```python
from build123d import *

# Parameters (mm, degrees)
SKETCH_1_W          = 95.5
SKETCH_1_H          = 95.5
EXTRUDE_1_DEPTH     = 7
CUT_EXTRUDE_1_DEPTH = 68.890536896
FILLET_2_R          = 15
SKETCH_3_R          = 75
EXTRUDE_2_DEPTH     = 2
CHAMFER_1_SIZE      = 7
FILLET_1_R          = 1
SKETCH_5_R          = 1.6
CUT_EXTRUDE_2_DEPTH = 107.296754489
SKETCH_6_W          = 42
SKETCH_6_H          = 42
CUT_EXTRUDE_3_DEPTH = 107.447170066
SKETCH_7_R          = 1.6
CUT_EXTRUDE_4_DEPTH = 107.447170066
CUT_EXTRUDE_5_DEPTH = 107.447170066
CUT_EXTRUDE_6_DEPTH = 0.5
SKETCH_10_W         = 12
SKETCH_10_H         = 12
CUT_EXTRUDE_7_DEPTH = 107.447170066
SKETCH_11_W         = 42
SKETCH_11_H         = 42
EXTRUDE_4_DEPTH     = 9
FILLET_3_R          = 2
SKETCH_12_W         = 41.3
SKETCH_12_H         = 41.3
CUT_EXTRUDE_8_DEPTH = 107.447170066
FILLET_4_R          = 5
SKETCH_13_R         = 3.25
CUT_EXTRUDE_9_DEPTH = 2


with BuildPart() as part:
    # ｽｹｯﾁ1 → ﾎﾞｽ - 押し出し1 (new body)
    with BuildSketch(Plane.XY):
        Rectangle(SKETCH_1_W, SKETCH_1_H)
    extrude(amount=EXTRUDE_1_DEPTH)

    # ｽｹｯﾁ2 → ｶｯﾄ - 押し出し1 (cut, through all)
    with BuildSketch(Plane.XY.offset(7)):
        Polygon((-16, 47.75), (-20, 20), (-47.75, 16), (-47.75, 47.75), align=None)
        Polygon((-16, -47.75), (-20, -20), (-47.75, -16), (-47.75, -47.75), align=None)
    cut_extrude_1 = extrude(amount=-CUT_EXTRUDE_1_DEPTH, mode=Mode.SUBTRACT)

    # ﾐﾗｰ1: ｶｯﾄ - 押し出し1 across plane
    add(cut_extrude_1.mirror(Plane(origin=(0, 0, 0), x_dir=(0, 0, 1), z_dir=(1, 0, 0))), mode=Mode.SUBTRACT)

    # ﾌｨﾚｯﾄ2
    fillet_2_edges = [part.edges().sort_by_distance(p)[0] for p in [
        (-20, 20, 3.5),
        (-20, -20, 3.5),
        (20, 20, 3.5),
        (20, -20, 3.5),
    ]]
    fillet(fillet_2_edges, radius=FILLET_2_R)

    # ｽｹｯﾁ3 → ﾎﾞｽ - 押し出し2 (add)
    with BuildSketch(Plane(origin=(0, 0, 0), x_dir=(-1, 0, 0), z_dir=(0, 0, -1))):
        Circle(SKETCH_3_R)
    extrude(amount=EXTRUDE_2_DEPTH)

    # 面取り1
    chamfer_1_edges = [part.edges().sort_by_distance(p)[0] for p in [
        (0, 47.75, 0),
        (47.75, 0, 0),
        (0, -47.75, 0),
        (-47.75, 0, 0),
    ]]
    chamfer(chamfer_1_edges, length=CHAMFER_1_SIZE - 0.0001)  # a hair under: the kernel refuses the full size

    # ﾌｨﾚｯﾄ1
    fillet_1_edges = [part.edges().sort_by_distance(p)[0] for p in [
        (75, 0, 0),
        (75, 0, -2),
    ]]
    fillet(fillet_1_edges, radius=FILLET_1_R - 0.0001)  # a hair under: the kernel refuses the full size

    # ｽｹｯﾁ5 → ｶｯﾄ - 押し出し2 (cut, through all)
    with BuildSketch(Plane.XY):
        with Locations((-34.25, 34.25)):
            Circle(SKETCH_5_R)
        with Locations((34.25, 34.25)):
            Circle(SKETCH_5_R)
        with Locations((34.25, -34.25)):
            Circle(SKETCH_5_R)
        with Locations((-34.25, -34.25)):
            Circle(SKETCH_5_R)
    extrude(amount=-CUT_EXTRUDE_2_DEPTH, mode=Mode.SUBTRACT)

    # ｽｹｯﾁ6 → ｶｯﾄ - 押し出し3 (cut, through all)
    with BuildSketch(Plane.XY.offset(7)):
        Rectangle(SKETCH_6_W, SKETCH_6_H)
    extrude(amount=-CUT_EXTRUDE_3_DEPTH, mode=Mode.SUBTRACT)

    # ｽｹｯﾁ7 → ｶｯﾄ - 押し出し4 (cut, through all)
    with BuildSketch(Plane.XY.offset(7)):
        with Locations((0, 37.75)):
            Circle(SKETCH_7_R)
        with Locations((-37.75, 0)):
            Circle(SKETCH_7_R)
        with Locations((37.75, 0)):
            Circle(SKETCH_7_R)
        with Locations((0, -37.75)):
            Circle(SKETCH_7_R)
    extrude(amount=-CUT_EXTRUDE_4_DEPTH, mode=Mode.SUBTRACT)

    # ｽｹｯﾁ8 → ｶｯﾄ - 押し出し5 (cut, through all)
    with BuildSketch(Plane(origin=(0, 0, -2), x_dir=(-1, 0, 0), z_dir=(0, 0, -1))):
        Polygon((-47.54163056, 53.19848481), (-45.04163056, 50.69848481), (-43.980970389, 51.759144982), (-46.480970389, 54.259144982), align=None)
        Polygon((-53.19848481, 47.54163056), (-54.259144982, 46.480970389), (-51.759144982, 43.980970389), (-50.69848481, 45.04163056), align=None)
        Polygon((45.748737342, 53.526911935), (43.980970389, 51.759144982), (45.04163056, 50.69848481), (46.809397513, 52.466251763), align=None)
        Polygon((52.466251763, 46.809397513), (50.69848481, 45.04163056), (51.759144982, 43.980970389), (53.526911935, 45.748737342), align=None)
    cut_extrude_5 = extrude(amount=-CUT_EXTRUDE_5_DEPTH, mode=Mode.SUBTRACT)

    # ｽｹｯﾁ9 → ｶｯﾄ - 押し出し6 (cut)
    with BuildSketch(Plane.XY):
        Polygon((-53.526911935, 45.748737342), (-45.748737342, 53.526911935), (-43.980970389, 51.759144982), (-51.759144982, 43.980970389), align=None)
        Polygon((46.480970389, 54.259144982), (43.980970389, 51.759144982), (51.759144982, 43.980970389), (54.259144982, 46.480970389), align=None)
    cut_extrude_6 = extrude(amount=-CUT_EXTRUDE_6_DEPTH, mode=Mode.SUBTRACT)

    # ﾐﾗｰ2: ｶｯﾄ - 押し出し5, ｶｯﾄ - 押し出し6 across plane
    add(cut_extrude_5.mirror(Plane.ZX), mode=Mode.SUBTRACT)
    add(cut_extrude_6.mirror(Plane.ZX), mode=Mode.SUBTRACT)

    # ｽｹｯﾁ10 → ｶｯﾄ - 押し出し7 (cut, through all)
    with BuildSketch(Plane.XY.offset(7)):
        with Locations((-29.75, -9.25)):
            Rectangle(SKETCH_10_W, SKETCH_10_H)
        with Locations((-9.25, 29.75)):
            Rectangle(SKETCH_10_W, SKETCH_10_H)
        with Locations((29.75, 9.25)):
            Rectangle(SKETCH_10_W, SKETCH_10_H)
        with Locations((9.25, -29.75)):
            Rectangle(SKETCH_10_W, SKETCH_10_H)
    extrude(amount=-CUT_EXTRUDE_7_DEPTH, mode=Mode.SUBTRACT)

    # ｽｹｯﾁ11 → ﾎﾞｽ - 押し出し4 (add, through all)
    with BuildSketch(Plane(origin=(0, 0, -2), x_dir=(-1, 0, 0), z_dir=(0, 0, -1))):
        Rectangle(SKETCH_11_W, SKETCH_11_H)
    extrude(amount=-EXTRUDE_4_DEPTH)

    # ﾌｨﾚｯﾄ3
    fillet_3_edges = [part.edges().sort_by_distance(p)[0] for p in [
        (-35.75, -15.25, 2.5),
        (-35.75, -3.25, 2.5),
        (-23.75, -3.25, 2.5),
        (-23.75, -15.25, 2.5),
        (-15.25, 23.75, 2.5),
        (-15.25, 35.75, 2.5),
        (-3.25, 35.75, 2.5),
        (-3.25, 23.75, 2.5),
        (23.75, 3.25, 2.5),
        (23.75, 15.25, 2.5),
        (35.75, 15.25, 2.5),
        (35.75, 3.25, 2.5),
        (15.25, -23.75, 2.5),
        (15.25, -35.75, 2.5),
        (3.25, -35.75, 2.5),
        (3.25, -23.75, 2.5),
    ]]
    fillet(fillet_3_edges, radius=FILLET_3_R)

    # ｽｹｯﾁ12 → ｶｯﾄ - 押し出し8 (cut, through all)
    with BuildSketch(Plane.XY.offset(7)):
        Rectangle(SKETCH_12_W, SKETCH_12_H)
    extrude(amount=-CUT_EXTRUDE_8_DEPTH, mode=Mode.SUBTRACT)

    # ﾌｨﾚｯﾄ4
    fillet_4_edges = [part.edges().sort_by_distance(p)[0] for p in [
        (-20.65, -20.65, 2.5),
        (-20.65, 20.65, 2.5),
        (20.65, 20.65, 2.5),
        (20.65, -20.65, 2.5),
    ]]
    fillet(fillet_4_edges, radius=FILLET_4_R)

    # ｽｹｯﾁ13 → ｶｯﾄ - 押し出し9 (cut)
    with BuildSketch(Plane(origin=(0, 0, -2), x_dir=(-1, 0, 0), z_dir=(0, 0, -1))):
        with Locations((-37.75, 0)):
            Circle(SKETCH_13_R)
        with Locations((0, -37.75)):
            Circle(SKETCH_13_R)
        with Locations((37.75, 0)):
            Circle(SKETCH_13_R)
        with Locations((0, 37.75)):
            Circle(SKETCH_13_R)
    extrude(amount=-CUT_EXTRUDE_9_DEPTH, mode=Mode.SUBTRACT)


solid = part.part
```
Read the model definition and answer for the solid it produces. Units are mm, in the model's axes. A direction names the side the tool comes from. Coordinates: 2 decimals unless noted, no trailing zeros. Return JSON: item names as keys, results as strings.
Item 1: Find section A-A (z = 5). Count the separate pieces of the cut face and the enclosed holes in it, plus the area to 3 significant figures.
Answers:
{"separate pieces": "1", "enclosed holes": "9", "area": "3,670 mm2"}
Item 2: For faces 4 (the flat face through (-35.75, -9, 3)), 5 (the flat face through (-49, -49, -0.5)), 6 (the cylindrical face through (34.748, -1.245, -1.014)), determine the directions among +Z, -Z, +X, -X, +Y, -Y from which every point of the face is accessible in a straight line to the end or side of a thin tool.
Answers:
{"face 4": "+Z, -Z", "face 5": "+Z", "face 6": "-Z"}
Item 3: Find the intervals of material crossed by probe 1 along Y at (x, z) = (0, -0.7); probe 2 along Y at (x, z) = (0, 4.5); probe 3 along Z at (x, y) = (35, -50), in increasing order.
Answers:
{"probe 1": "y = -74.95 to -41, -34.5 to -20.65, 20.65 to 34.5, 41 to 74.95", "probe 2": "y = -50.25 to -39.35, -36.15 to -20.65, 20.65 to 36.15, 39.35 to 50.25", "probe 3": "z = -2 to 0"}
Item 4: Flat-ended cylindrical pins translate along their axes: P1, Ø6, axis at x = -49, y = -48.5, coming from the +Z side; P2, Ø2.5, axis at y = -10.5, z = 4, coming from the +X side; P3, Ø3.5, axis at x = 0, y = 37.75, coming from the -Z side; P4, Ø5, axis at x = 1.5, y = -38.5, coming from the -Z side. Find the tip coordinate at first contact, or state that the pin passes through.
Answers:
{"P1": "stops at z = 0", "P2": "stops at x = 52", "P3": "stops at z = 0", "P4": "stops at z = -2"}
Item 5: For a pull along X with two mould halves and no side action, classify faces 1 (the flat face through (40.135, -17.098, 3.549)), 2 (the flat face through (-0.22, 51.2, 3.55)), 3 (the cylindrical face through (36.57, 1.08, 3.55)) as +X half, -X half, draft (parallel to the pull), parting line (faces both ways), or undercut.
Answers:
{"face 1": "+X half", "face 2": "draft", "face 3": "undercut"}
